Read the model definition and answer for the solid it produces. Units are mm, in the model's axes. Give positions to 0.01 mm unless a question says otherwise; leave off trailing zeros. Loops run counter-clockwise (first coordinate to the right, second up) from the corner with the lowest first, then second, coordinate; pieces in that order, holes last.
(1) Find section A-A, the plane z = 0. Write down the section's boundary in (x, y).
(2) Each of these flat-tipped pins is pushed along its axis until it touches: P1, Ø3, axis at x = -11.84, z = 20.5, coming from the -Y side; P2, Ø1.5, axis at x = -11.5, y = 2, coming from the -Z side. Where does it stop, or does it pass through?
(3) Find section C-C, the plane z = -10.5. Write down the section's boundary in (x, y).
(4) Find section D-D, the plane y = 2.5. Write down the section's boundary in (x, z).
(5) Determine the mould class of faces 1 (the face through (-24.16, 2, 0)), 2 (the face through (-12.183, 2.028, 22.063)), 3 (the face through (26.62, 1.97, 1.01)) for opening direction Z: pulls with the +Z half, pulls with the -Z half, needs draft (parallel to the pull), parting line crosses it, or undercut.
(6) Find section B-B, the plane x = 0. Write down the section's boundary in (y, z).
(7) Straight lines are drawn through the part: probe 1 along X at (y, z) = (0.8, 0); probe 2 along X at (y, z) = (0.6, 16); probe 3 along X at (y, z) = (0.5, -4.5). For each, find the intervals that lie inside material, in ascending order.
```python
from build123d import *

# Parameters (mm, degrees)
SKETCH_1_R               = 26.64
EXTRUDE_1_DEPTH          = 4
SKETCH_2_R               = 21.25
CUT_EXTRUDE_1_DEPTH      = 4
SKETCH_3_R               = 1.6
CUT_EXTRUDE_2_DEPTH      = 4
PATTERN_CIRCULAR_1_COUNT = 3
SKETCH_5_W               = 17.203489066
SKETCH_5_H               = 59.100654928
CUT_EXTRUDE_3_DEPTH      = 4


with BuildPart() as part:
    # 草图1 → 凸台-拉伸1 (new body)
    with BuildSketch(Plane(origin=(0, 0, 0), x_dir=(1, 0, 0), z_dir=(0, 1, 0))):
        Circle(SKETCH_1_R)
    extrude(amount=EXTRUDE_1_DEPTH)

    # 草图2 → 切除-拉伸1 (cut)
    with BuildSketch(Plane(origin=(0, 4, 0), x_dir=(1, 0, 0), z_dir=(0, 1, 0))):
        Circle(SKETCH_2_R)
    extrude(amount=-CUT_EXTRUDE_1_DEPTH, mode=Mode.SUBTRACT)

    # 草图3 → 切除-拉伸2 (cut)
    with BuildSketch(Plane(origin=(0, 4, 0), x_dir=(1, 0, 0), z_dir=(0, 1, 0))):
        with Locations((23.672055427, 0)):
            Circle(SKETCH_3_R)
    cut_extrude_2 = extrude(amount=-CUT_EXTRUDE_2_DEPTH, mode=Mode.SUBTRACT)

    # 阵列(圆周)1: 切除-拉伸2 ×3 about axis
    pattern_circular_1_axis = Axis((0, 0, 0), (0, 1, 0))
    for i in range(1, PATTERN_CIRCULAR_1_COUNT):
        add(cut_extrude_2.rotate(pattern_circular_1_axis, i * 360 / PATTERN_CIRCULAR_1_COUNT), mode=Mode.SUBTRACT)

    # 草图5 → 切除-拉伸3 (cut)
    with BuildSketch(Plane(origin=(0, 4, 0), x_dir=(1, 0, 0), z_dir=(0, 1, 0))):
        with Locations((-32.761744533, -1.256680407)):
            Rectangle(SKETCH_5_W, SKETCH_5_H)
    extrude(amount=-CUT_EXTRUDE_3_DEPTH, mode=Mode.SUBTRACT)


solid = part.part
```
Entries:
1. outline: (-24.16, 0) - (-21.25, 0) - (-21.25, 4) - (-24.16, 4) - close; (21.25, 0) - (22.07, 0) - (22.07, 4) - (21.25, 4) - close; (25.27, 0) - (26.64, 0) - (26.64, 4) - (25.27, 4) - close
2. P1: passes through
2. P2: stops at z = -24.37
3. outline: (-24.16, 0) - (-18.47, 0) - (-18.47, 4) - (-24.16, 4) - close; (18.47, 0) - (24.48, 0) - (24.48, 4) - (18.47, 4) - close
4. outline: (-24.16, -11.22) arc R26.64 ccw (long way) to (-24.16, 11.22) - close; hole circle Ø42.5 at (0, 0); hole circle Ø3.2 at (-11.84, -20.5); hole circle Ø3.2 at (-11.84, 20.5); hole circle Ø3.2 at (23.67, 0)
5. face 1: needs draft
5. face 2: undercut
5. face 3: parting line crosses it
6. outline: (0, -26.64) - (4, -26.64) - (4, -21.25) - (0, -21.25) - close; (0, 21.25) - (4, 21.25) - (4, 26.64) - (0, 26.64) - close
7. probe 1: x = -24.16 to -21.25, 21.25 to 22.07, 25.27 to 26.64
7. probe 2: x = -21.3 to -13.98, 13.98 to 21.3
7. probe 3: x = -24.16 to -20.77, 20.77 to 26.26
